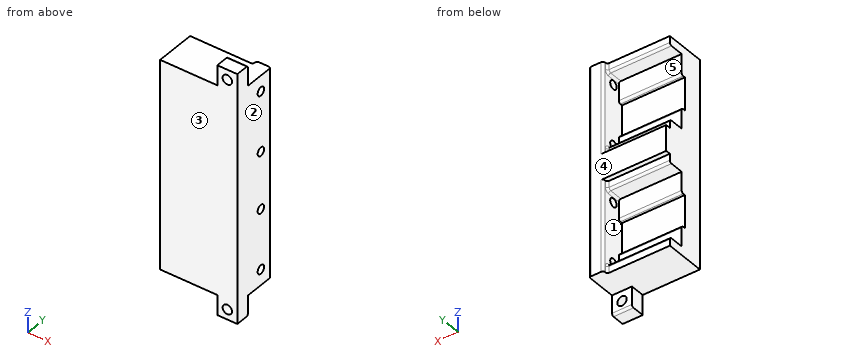
from build123d import *

# Parameters (mm, degrees)
BOSS_EXTRUDE1_DEPTH = 11
SKETCH3_W           = 22
SKETCH3_H           = 3
BOSS_EXTRUDE2_DEPTH = 14
BOSS_EXTRUDE3_DEPTH = 5
SKETCH5_R           = 1.5
CUT_EXTRUDE1_DEPTH  = 36.096650541
SKETCH6_W           = 7
SKETCH6_H           = 7
BOSS_EXTRUDE4_DEPTH = 5
SKETCH10_R          = 1.65
CUT_EXTRUDE2_DEPTH  = 33.123192233
SKETCH8_W           = 27
SKETCH8_H           = 15.7
BOSS_EXTRUDE5_DEPTH = 4.5
FILLET1_R           = 0.75


with BuildPart() as part:
    # Sketch1 → Boss-Extrude1 (new, symmetric)
    with BuildSketch(Plane(origin=(0, 0, 0), x_dir=(0, 0, -1), z_dir=(1, 0, 0))):
        Polygon((-13.0089, 0), (13.0089, 0), (13.0089, 8.5), (5.7589, 8.5), (5.7589, 7), (-5.7589, 7), (-5.7589, 8.5), (-13.0089, 8.5), align=None)
    extrude(amount=BOSS_EXTRUDE1_DEPTH, both=True)

    # Sketch3 → Boss-Extrude2 (add)
    with BuildSketch(Plane.XZ):
        with Locations((0, -14.5089)):
            Rectangle(SKETCH3_W, SKETCH3_H)
        with Locations((0, 14.5089)):
            Rectangle(SKETCH3_W, SKETCH3_H)
    extrude(amount=-BOSS_EXTRUDE2_DEPTH)

    # Sketch4 → Boss-Extrude3 (add)
    with BuildSketch(Plane(origin=(11, 0, 0), x_dir=(0, 0, -1), z_dir=(1, 0, 0))):
        Polygon((-8.8, 15.7), (-16.0089, 15.7), (-16.0089, 0), (16.0089, 0), (16.0089, 15.7), align=None)
    extrude(amount=BOSS_EXTRUDE3_DEPTH)

    # Sketch5 → Cut-Extrude1 (cut, through all)
    with BuildSketch(Plane(origin=(16, 0, 0), x_dir=(0, 0, -1), z_dir=(1, 0, 0))):
        with Locations((-10.5, 11)):
            Circle(SKETCH5_R)
        with Locations((10.5, 11)):
            Circle(SKETCH5_R)
    extrude(amount=-CUT_EXTRUDE1_DEPTH, mode=Mode.SUBTRACT)

    # Sketch6 → Boss-Extrude4 (add)
    with BuildSketch(Plane.XZ):
        with Locations((12.5, 19.5089)):
            Rectangle(SKETCH6_W, SKETCH6_H)
    extrude(amount=-BOSS_EXTRUDE4_DEPTH)

    # Sketch10 → Cut-Extrude2 (cut, through all)
    with BuildSketch(Plane.XZ):
        with Locations(Location((12.5, 19.5089, 0), (0, 0, 270))):
            Circle(SKETCH10_R)
    extrude(amount=-CUT_EXTRUDE2_DEPTH, mode=Mode.SUBTRACT)

    # Sketch8 → Boss-Extrude5 (add)
    with BuildSketch(Plane(origin=(0, 0, -16.0089), x_dir=(-1, 0, 0), z_dir=(0, 0, -1))):
        with Locations((-2.5, 7.85)):
            Rectangle(SKETCH8_W, SKETCH8_H)
    extrude(amount=BOSS_EXTRUDE5_DEPTH)

    # Fillet1
    fillet1_edges = [part.edges().sort_by_distance(p)[0] for p in [
        (0, 8.5, 5.7589),
        (0, 8.5, -5.7589),
        (0, 14, -13.0089),
        (11, 14, -14.5089),
        (11, 11.25, -13.0089),
        (11, 14, 14.5089),
        (11, 11.25, 13.0089),
        (0, 14, 13.0089),
        (11, 15.7, 0),
        (16, 15.7, -2.25),
        (12.5, 5, 23.0089),
    ]]
    fillet(fillet1_edges, radius=FILLET1_R)

    # Mirror6: part across plane


with BuildPart() as part_1:
    add(part.part)
    add(part.part.mirror(Plane(origin=(0, 0, -20.5089), x_dir=(1, 0, 0), z_dir=(0, 0, -1))))


solid = part_1.part
Here's how the part is built. I have some questions about the finished solid (model axes, mm). Face numbers are marked on the shaded views. A direction names the side the tool comes from. Give positions to 0.01 mm unless a question says otherwise; leave off trailing zeros. Order: outer loops, then holes, each group sorted by start corner. A loop starts at its lowest first (then second) coordinate and runs counter-clockwise, first axis right, second up. Notation, with made-up numbers: M -16,78 L 29,78 A19 ccw 29,107 Z; hole C 59,25.25 d2. An arc over 180 degrees is marked long. Answer as a JSON object with one key per item and string values. Group by question number.
1) Suppose I cut it at C-C, the plane y = 11. Count the separate pieces of the cut face and the enclosed holes in it, plus the area to 3 significant figures.
2) Suppose I cut it at B-B, the plane z = -10.5. Write out the boundary of the cut face in (x, y).
3) I'm going to push flat-ended pins straight in: pin 1 Ø2 at (x, z) = (3, -8.5) entering from +Y; pin 2 Ø3.5 at (y, z) = (11, -51.52) entering from -X; pin 3 Ø1.4 at (x, y) = (2.5, 11) entering from -Z. Where does each tip first touch, or does it pass through?
4) Please list where these lines run through material, in increasing order: L1, parallel to Z at x = 2.75, y = 11.75; L2, parallel to Y at x = 13.15, z = -10.5; L3, parallel to Y at x = -3, z = 2. Write a range as [from, to].
5) We'd pull the mould along X, two halves only. Please class the marked faces 1, 2 and 3: pulls with the +X half, pulls with the -X half, needs draft (parallel to the pull), parting line crosses it, or undercut.
6) Suppose I cut it at D-D, the plane y = 1.75. Write out the boundary of the cut face in (x, z).
7) On a 3-axis mill with a long thin cutter (end or side, diameter ignored), from which of +Z, -Z, +X, -X, +Y, -Y can I reach the whole of each face in a straight line? I mean the marked faces 4 and 5. Say none if no direction works.
8) Suppose I cut it at A-A, the plane x = 12.5. Write out the boundary of the cut face in (y, z).
Results found:
{
 "1": {"separate pieces": "5", "enclosed holes": "0", "area": "768 mm²"},
 "2": {"outline": "M -11,0 L 16,0 L 16,9.5 L 11,9.5 L 11,8.5 L -11,8.5 Z; M 11,12.5 L 16,12.5 L 16,14.95 A0.75 ccw 15.25,15.7 L 11.75,15.7 A0.75 ccw 11,14.95 Z"},
 "3": {"pin 1": "y = 8.5", "pin 2": "x = 11", "pin 3": "z = -57.03"},
 "4": {"L1": "[-57.03, -54.03], [-28.01, -13.01], [13.01, 16.01]", "L2": "[0, 9.5], [12.5, 15.7]", "L3": "[0, 7]"},
 "5": {"face 1": "pulls with the -X half", "face 2": "pulls with the +X half", "face 3": "needs draft"},
 "6": {"outline": "M -11,-57.03 L 9,-57.03 L 9,-64.03 L 16,-64.03 L 16,23.01 L 9,23.01 L 9,16.01 L -11,16.01 Z; hole C 12.5,-60.53 d3.3; hole C 12.5,19.51 d3.3"},
 "7": {"face 4": "+Z, -Z, +X, -X, +Y", "face 5": "-X, +Y"},
 "8": {"outline": "M 0,-64.03 L 4.25,-64.03 A0.75 ccw 5,-63.28 L 5,-62.18 L 0,-62.18 Z; M 0,-58.88 L 5,-58.88 L 5,-57.03 L 15.7,-57.03 L 15.7,16.01 L 5,16.01 L 5,17.86 L 0,17.86 Z; M 0,21.16 L 5,21.16 L 5,22.26 A0.75 ccw 4.25,23.01 L 0,23.01 Z; hole C 11,-51.52 d3; hole C 11,-30.52 d3; hole C 11,-10.5 d3; hole C 11,10.5 d3"}
}
